```python
from build123d import *

# Parameters (mm, degrees)
EXTRUDE1_DEPTH = 2.54
CHAMFER1_SIZE  = 1.27


with BuildPart() as part:
    # Sketch1 → Extrude1 (new body, symmetric)
    with BuildSketch(Plane.XY):
        Polygon((0, 63.5), (42.121134838, 0), (0, 0), align=None)
    extrude(amount=EXTRUDE1_DEPTH, both=True)

    # Chamfer1
    chamfer1_edges = [part.edges().sort_by_distance(p)[0] for p in [
        (21.060567419, 31.75, 2.54),
        (21.060567419, 31.75, -2.54),
        (21.060567419, 0, -2.54),
        (21.060567419, 0, 2.54),
    ]]
    chamfer(chamfer1_edges, length=CHAMFER1_SIZE)


solid = part.part
```
For this review, take the finished solid that the model builds, in its own axes (mm). Round coordinates to 2 decimals unless told otherwise and drop trailing zeros. Write each loop counter-clockwise with the first axis right and the second up, starting at its lowest first coordinate (ties: lowest second). Pieces come first, ordered by that corner, then holes. Notation, with made-up numbers: (-22.5, 11) - (-13.5, 11) arc R20 cw to (-13.5, 17) - close; hole circle Ø7 at (50, 76). An arc over 180 degrees is marked (long way). Answer as a JSON object with one key per item and string values.
1. We need section C-C on y = 5.5. Give the boundary of the cut face in (x, z).
Response values:
{"outline": "(0, -2.54) - (36.95, -2.54) - (38.47, -1.27) - (38.47, 1.27) - (36.95, 2.54) - (0, 2.54) - close"}
2. We need section A-A on x = 13. Give the boundary of the cut face in (y, z), then the cut area to 3 significant figures.
Response values:
{"outline": "(0, -1.27) - (1.27, -2.54) - (41.6, -2.54) - (43.9, -1.27) - (43.9, 1.27) - (41.6, 2.54) - (1.27, 2.54) - (0, 1.27) - close", "area": "218 mm2"}
3. We need section B-B on z = 0.55. Give the boundary of the cut face in (x, y), then the cut area to 3 significant figures.
Response values:
{"outline": "(0, 0) - (42.12, 0) - (0, 63.5) - close", "area": "1,340 mm2"}
4. We need section D-D on x = 4.5. Give the boundary of the cut face in (y, z), then the cut area to 3 significant figures.
Response values:
{"outline": "(0, -1.27) - (1.27, -2.54) - (54.42, -2.54) - (56.72, -1.27) - (56.72, 1.27) - (54.42, 2.54) - (1.27, 2.54) - (0, 1.27) - close", "area": "284 mm2"}
5. For pin 1 Ø5 at (x, y) = (24.5, 26) entering from +Z; pin 2 Ø2 at (y, z) = (18.5, 0) entering from +X; pin 3 Ø3 at (x, y) = (16.5, 44) entering from -Z; pin 4 Ø3 at (y, z) = (31, 0.5) entering from +X, all flat-tipped, find the tip position at first contact; note any pin that passes through.
Response values:
{"pin 1": "stops at z = 2.54", "pin 2": "stops at x = 30.51", "pin 3": "passes through", "pin 4": "stops at x = 22.55"}
6. To check wall thickness, follow line 1 along X through (y, z) = (13, -2.25); line 2 along X through (y, z) = (36, -0.1); line 3 along Y through (x, z) = (35, 1.25). State the ranges of each line that lie inside material, in increasing order.
Response values:
{"line 1": "x = 0 to 32.32", "line 2": "x = 0 to 18.24", "line 3": "y = 0 to 10.74"}
